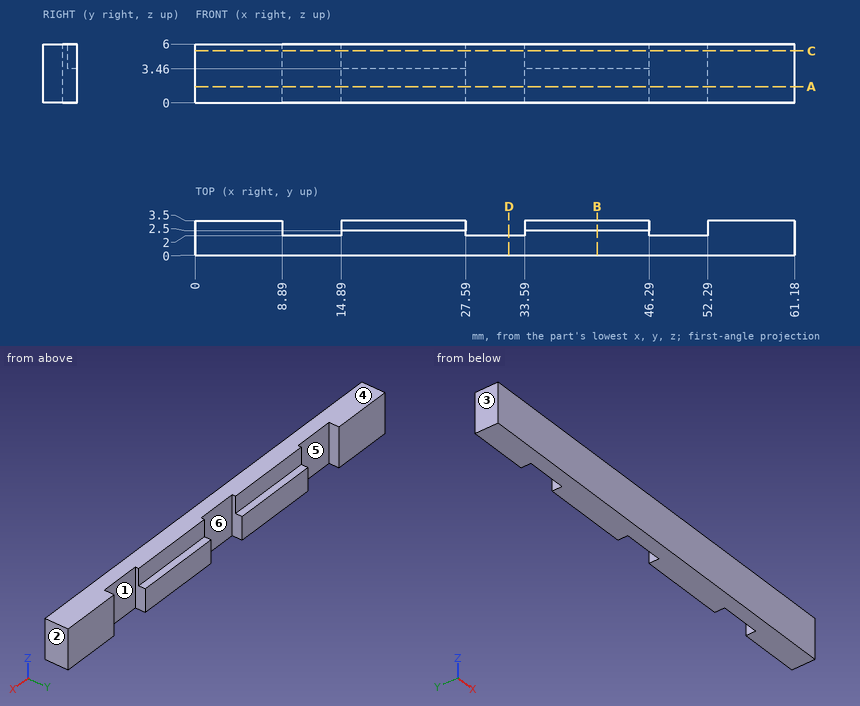
For this review, use the dimensioned drawing (mm, ordinates from the lowest corner) and the shaded views. A direction names the side the tool comes from. Give positions to 0.01 mm unless a question says otherwise; leave off trailing zeros. Loops run counter-clockwise (first coordinate to the right, second up) from the corner with the lowest first, then second, coordinate; pieces in that order, holes last.
Item 1: Take a section at C-C, the plane z = 5.3. State the section outline as (x, y) points.
Item 2: Tool access review of the marked faces 1 and 2: name each direction out of +Z, -Z, +X, -X, +Y, -Y from which nothing blocks a thin tool from reaching the whole face with its end or side.
Item 3: For line 1 along X through (y, z) = (2.9, 2.95); line 2 along X through (y, z) = (2.7, 4.55); line 3 along Z through (x, y) = (43.5, 2.7), list the stretches that pass through material, from the lowest coordinate up.
Item 4: Take a section at A-A, the plane z = 1.65. State the section outline as (x, y) points.
Item 5: Draft analysis for pull direction X (two halves, no side actions). For the marked faces 3, 4, 5 and 6, state which applies: +X half, -X half, draft (parallel to the pull), parting line (faces both ways), or undercut.
Item 6: Take a section at D-D, the plane x = 32. State the section outline as (y, z) points, and give its area (3 significant figures).
Item 7: Insertion check: pin 1 (1.5 mm diameter, centred on x = 13.5, z = 2.5, fed in from +Y). The pin has a flat end and moves straight along its axis. Give the tip position at first contact, or say it passes through.
Item 8: Take a section at B-B, the plane x = 41. State the section outline as (y, z) points.
Calculated:
1. outline: (0, 0) - (61.18, 0) - (61.18, 3.5) - (52.29, 3.5) - (52.29, 2) - (46.29, 2) - (46.29, 2.5) - (33.59, 2.5) - (33.59, 2) - (27.59, 2) - (27.59, 2.5) - (14.89, 2.5) - (14.89, 2) - (8.89, 2) - (8.89, 3.5) - (0, 3.5) - close
2. face 1: +Z, -Z, +Y
2. face 2: +Z, -Z, +X, +Y, -Y
3. line 1: x = 0 to 8.89, 14.89 to 27.59, 33.59 to 46.29, 52.29 to 61.18
3. line 2: x = 0 to 8.89, 52.29 to 61.18
3. line 3: z = 0 to 3.46
4. outline: (0, 0) - (61.18, 0) - (61.18, 3.5) - (52.29, 3.5) - (52.29, 2) - (46.29, 2) - (46.29, 3.5) - (33.59, 3.5) - (33.59, 2) - (27.59, 2) - (27.59, 3.5) - (14.89, 3.5) - (14.89, 2) - (8.89, 2) - (8.89, 3.5) - (0, 3.5) - close
5. face 3: -X half
5. face 4: draft
5. face 5: undercut
5. face 6: undercut
6. outline: (0, 0) - (2, 0) - (2, 6) - (0, 6) - close
6. area: 12.0 mm2
7. pin 1: stops at y = 2
8. outline: (0, 0) - (3.5, 0) - (3.5, 3.46) - (2.5, 3.46) - (2.5, 6) - (0, 6) - close
